The model under review builds one solid part; all positions refer to its coordinate system, in mm. Face numbers are marked on the shaded views. A direction names the side the tool comes from. Coordinates: 2 decimals unless noted, no trailing zeros. Write each loop counter-clockwise with the first axis right and the second up, starting at its lowest first coordinate (ties: lowest second). Pieces come first, ordered by that corner, then holes.
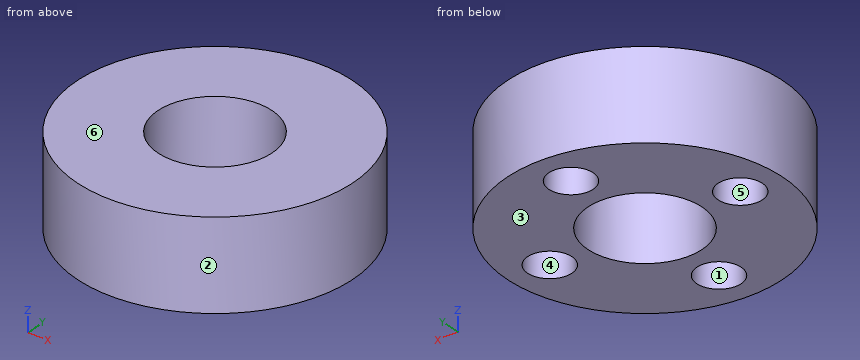
```python
from build123d import *

# Parameters (mm, degrees)
SKETCH2_R           = 10.85
SKETCH2_R_2         = 1.75
SKETCH2_R_3         = 4.5
BOSS_EXTRUDE1_DEPTH = 7
SKETCH3_R           = 1.75
BOSS_EXTRUDE2_DEPTH = 3


with BuildPart() as part:
    # Sketch2 → Boss-Extrude1 (new body)
    with BuildSketch(Plane.XY.offset(-31.892451267)):
        Circle(SKETCH2_R)
        with Locations((-7.6, 0)):
            Circle(SKETCH2_R_2, mode=Mode.SUBTRACT)
        with Locations((7.6, 0)):
            Circle(SKETCH2_R_2, mode=Mode.SUBTRACT)
        Circle(SKETCH2_R_3, mode=Mode.SUBTRACT)
        with Locations((0, 7.6)):
            Circle(SKETCH2_R_2, mode=Mode.SUBTRACT)
        with Locations((0, -7.6)):
            Circle(SKETCH2_R_2, mode=Mode.SUBTRACT)
    extrude(amount=BOSS_EXTRUDE1_DEPTH)

    # Sketch3 → Boss-Extrude2 (add)
    with BuildSketch(Plane.XY.offset(-24.892451267)):
        with Locations((0, 7.6)):
            Circle(SKETCH3_R)
        with Locations((-7.6, 0)):
            Circle(SKETCH3_R)
        with Locations((0, -7.6)):
            Circle(SKETCH3_R)
        with Locations((7.6, 0)):
            Circle(SKETCH3_R)
    extrude(amount=-BOSS_EXTRUDE2_DEPTH)


solid = part.part
```
Item 1: Mouldability with a two-part tool opening along X and no side actions: class the marked faces 1, 2, 3 and 4 as pulls with the +X half, pulls with the -X half, needs draft (parallel to the pull), parting line crosses it, or undercut.
Solved:
face 1: undercut
face 2: parting line crosses it
face 3: needs draft
face 4: undercut
Item 2: Take a section at A-A, the plane x = 0. Write out the cut boundary in (y, z).
Solved:
outline: (-10.85, -31.89) - (-9.35, -31.89) - (-9.35, -27.89) - (-5.85, -27.89) - (-5.85, -31.89) - (-4.5, -31.89) - (-4.5, -24.89) - (-10.85, -24.89) - close; (4.5, -31.89) - (5.85, -31.89) - (5.85, -27.89) - (9.35, -27.89) - (9.35, -31.89) - (10.85, -31.89) - (10.85, -24.89) - (4.5, -24.89) - close
Item 3: Take a section at D-D, the plane z = -25.25. Write out the cut boundary in (x, y), plus the area to 3 significant figures.
Solved:
outline: circle Ø21.7 at (0, 0); hole circle Ø9 at (0, 0)
area: 306 mm2
Item 4: To check wall thickness, follow line 1 along Y through (x, z) = (0, -30.3); line 2 along X through (y, z) = (-0.75, -30); line 3 along X through (y, z) = (-1.5, -28.25). State the ranges of each line that lie inside material, in increasing order.
Solved:
line 1: y = -10.85 to -9.35, -5.85 to -4.5, 4.5 to 5.85, 9.35 to 10.85
line 2: x = -10.82 to -9.18, -6.02 to -4.44, 4.44 to 6.02, 9.18 to 10.82
line 3: x = -10.75 to -8.5, -6.7 to -4.24, 4.24 to 6.7, 8.5 to 10.75
Item 5: Machinability: for the marked faces 5 and 6, which of the approach directions +Z, -Z, +X, -X, +Y, -Y give a long, thin tool a straight path to every point of the face, cutting with its end or side? Answer none if there is none.
Solved:
face 5: -Z
face 6: +Z, +X, -X, +Y, -Y
Item 6: For pin 1 (4 mm diameter, centred on x = -7, y = 0, fed in from -Z); pin 2 (2 mm diameter, centred on x = -7.6, y = 0, fed in from -Z); pin 3 (4 mm diameter, centred on x = 3, z = -29, fed in from +Y); pin 4 (1.5 mm diameter, centred on y = -2.5, z = -28.5, fed in from +X), all flat-tipped, find the tip position at first contact; note any pin that passes through.
Solved:
pin 1: stops at z = -31.89
pin 2: stops at z = -27.89
pin 3: stops at y = 10.8
pin 4: stops at x = 10.71
Item 7: Take a section at C-C, the plane z = -29.5. Write out the cut boundary in (x, y), plus the area to 3 significant figures.
Solved:
outline: circle Ø21.7 at (0, 0); hole circle Ø3.5 at (-7.6, 0); hole circle Ø9 at (0, 0); hole circle Ø3.5 at (0, -7.6); hole circle Ø3.5 at (0, 7.6); hole circle Ø3.5 at (7.6, 0)
area: 268 mm2
